Part model, mm, in its own coordinate system. A direction names the side the tool comes from. Round coordinates to 2 decimals unless told otherwise and drop trailing zeros. Write each loop counter-clockwise with the first axis right and the second up, starting at its lowest first coordinate (ties: lowest second). Pieces come first, ordered by that corner, then holes. Notation, with made-up numbers: M -2.5,-6.5 L 55.5,-6.5 A22 ccw 55.5,27.5 Z; hole C -15.5,48 d8. An arc over 180 degrees is marked long. One line per question, with ' | ' between items. Start each with the question number.
1) Saw through at A-A (y = 0). Give the number of separate pieces and of enclosed holes in the cut face, plus the area to 3 significant figures.
2) Saw through at D-D (x = 23.5). List the corners of the cut face in (y, z), plus the area to 3 significant figures.
3) Mould opens along Y. For faces 1 (the face through (-0.488, 21.304, 1.521)), 2 (the face through (-0.1, 16.3, -1)), 3 (the face through (26.327, -10.916, 3.944)) say: pulls with the +Y half, pulls with the -Y half, needs draft (parallel to the pull), parting line crosses it, or undercut.
4) Tool access for faces 4 (the face through (0, -19, 0)), 5 (the face through (-26.7, -2.4, 5.5)), 6 (the face through (25.646, 0.676, 1.521)): list every direction of +Z, -Z, +X, -X, +Y, -Y with a clear straight run to the whole face (end or side of a thin tool).
5) Wall check: probe 1 along Y at (x, z) = (0, 4.25); probe 2 along X at (y, z) = (2.5, 6.25); probe 3 along Z at (x, y) = (4.5, -19). Give the ranges that are in metal, low to high. Write a range as [from, to].
6) Saw through at C-C (z = 5.25). List the corners of the cut face in (x, y), plus the area to 3 significant figures.
7) Drop flat-ended pins along their axis: pin 1 Ø6.5 at (x, y) = (22.5, -2) entering from +Z; pin 2 Ø4 at (y, z) = (-6.5, 2) entering from -X; pin 3 Ø3 at (x, z) = (-7.5, 4.5) entering from -Y; pin 4 Ø2 at (x, z) = (-17, 2.5) entering from +Y. Give the stop position or say it passes through.
```python
from build123d import *

# Parameters (mm, degrees)
SKETCH_1_R          = 28.5
SKETCH_1_R_2        = 15
EXTRUDE_1_DEPTH     = 8
SKETCH_2_R          = 18.4
SKETCH_2_R_2        = 16.1
EXTRUDE_2_DEPTH     = 1
SKETCH_3_R          = 4
CUT_EXTRUDE_1_DEPTH = 5
SKETCH_4_R          = 2.25
CUT_EXTRUDE_2_DEPTH = 42.297699694


with BuildPart() as part:
    # 草图1 → 拉伸1 (new body)
    with BuildSketch(Plane.XY):
        Circle(SKETCH_1_R)
        Circle(SKETCH_1_R_2, mode=Mode.SUBTRACT)
    extrude(amount=EXTRUDE_1_DEPTH)

    # 草图2 → 拉伸2 (add)
    with BuildSketch(Plane(origin=(0, 0, 0), x_dir=(-1, 0, 0), z_dir=(0, 0, -1))):
        with Locations(Location((0, 0, 0), (0, 0, 180))):
            Circle(SKETCH_2_R)
        Circle(SKETCH_2_R_2, mode=Mode.SUBTRACT)
    extrude(amount=EXTRUDE_2_DEPTH)

    # 草图3 → 切除-拉伸1 (cut)
    with BuildSketch(Plane.XY.offset(8)):
        with Locations((0, 23.5)):
            Circle(SKETCH_3_R)
        with Locations((-23.5, 0)):
            Circle(SKETCH_3_R)
        with Locations((0, -23.5)):
            Circle(SKETCH_3_R)
        with Locations((23.5, 0)):
            Circle(SKETCH_3_R)
    extrude(amount=-CUT_EXTRUDE_1_DEPTH, mode=Mode.SUBTRACT)

    # 草图4 → 切除-拉伸2 (cut, through all)
    with BuildSketch(Plane.XY.offset(8)):
        with Locations((-23.5, 0)):
            Circle(SKETCH_4_R)
        with Locations((0, 23.5)):
            Circle(SKETCH_4_R)
        with Locations((23.5, 0)):
            Circle(SKETCH_4_R)
        with Locations((0, -23.5)):
            Circle(SKETCH_4_R)
    extrude(amount=-CUT_EXTRUDE_2_DEPTH, mode=Mode.SUBTRACT)


solid = part.part
```
Answer key:
1) separate pieces: 4 | enclosed holes: 0 | area: 114 mm2
2) outline: M -16.12,0 L -2.25,0 L -2.25,3 L -4,3 L -4,8 L -16.12,8 Z; M 2.25,0 L 16.12,0 L 16.12,8 L 4,8 L 4,3 L 2.25,3 Z | area: 204 mm2
3) face 1: undercut | face 2: needs draft | face 3: parting line crosses it
4) face 4: -Z | face 5: +Z | face 6: +Z, -Z
5) probe 1: y = [-28.5, -27.5], [-19.5, -15], [15, 19.5], [27.5, 28.5] | probe 2: x = [-28.39, -26.62], [-20.38, -14.79], [14.79, 20.38], [26.62, 28.39] | probe 3: z = [0, 8]
6) outline: C 0,0 d57; hole C -23.5,0 d8; hole C 0,0 d30; hole C 0,-23.5 d8; hole C 0,23.5 d8; hole C 23.5,0 d8 | area: 1,640 mm2
7) pin 1: stops at z = 8 | pin 2: stops at x = -28.14 | pin 3: stops at y = -27.86 | pin 4: stops at y = 23.58
